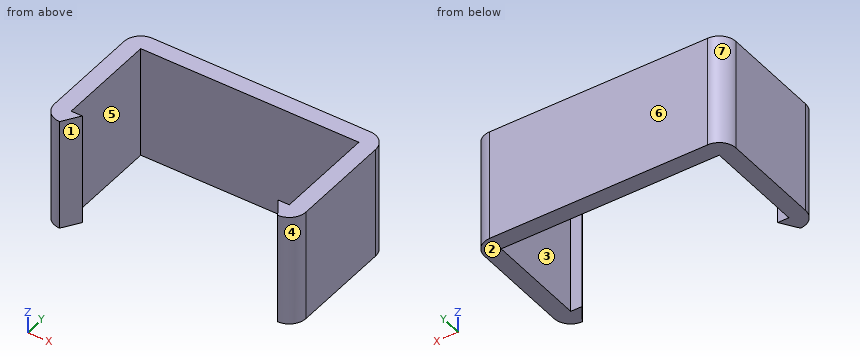
from build123d import *

# Parameters (mm, degrees)
F1_DEPTH = 20
F2_ANGLE = 270
F3_R     = 2.99999


# Not quite as in the source:
# - a fillet or chamfer is up to 0.001 mm smaller than in the source, because OpenCascade refuses the exact size


with BuildPart() as f1:
    # F0 (on Front) → F1 (new body)
    with BuildSketch(Plane.XZ):
        Polygon((22.5, 24), (-22.5, 24), (-22.5, 0), (-19.5, 0), (-17.5, 3), (-19.5, 3), (-19.5, 21), (19.5, 21), (19.5, 3), (17.5, 3), (19.5, 0), (22.5, 0), align=None)
    extrude(amount=F1_DEPTH)


with BuildPart() as f1_1:
    # F2: moved
    add(f1.part.rotate(Axis((0, -20, 24), (1, 0, 0)), F2_ANGLE))

    # F3 (radius 3 in the source; OpenCascade refuses exactly that, so slightly less here)
    f3_edges = [f1_1.edges().sort_by_distance(p)[0] for p in [
        (-22.5, -20, 14),
        (-22.5, -44, 14),
        (22.5, -44, 14),
        (22.5, -20, 14),
    ]]
    fillet(f3_edges, radius=F3_R)


solid = f1_1.part
Design review of the part built by this model. Coordinates are the model's own, in mm. Face numbers are marked on the shaded views. A direction names the side the tool comes from. Round coordinates to 2 decimals unless told otherwise and drop trailing zeros. Loops run counter-clockwise (first coordinate to the right, second up) from the corner with the lowest first, then second, coordinate; pieces in that order, holes last. Notation, with made-up numbers: (48.5, 86) -> (107.5, 86) arc R22 cw to (107.5, 122) -> close; hole circle Ø3 at (79.5, -39.75). An arc over 180 degrees is marked (long way). Use one line per item in the form item = value. Start each with the question number.
Q1. Draft analysis for pull direction X (two halves, no side actions). For the marked faces 4, 5, 6 and 7, state which applies: +X half, -X half, draft (parallel to the pull), parting line (faces both ways), or undercut.
Q2. For pin 1 Ø12 at (x, z) = (-2, 13) entering from -Y, flat-tipped, find the tip position at first contact; note if it passes through.
Q3. We need section A-A on y = -37. Give the boundary of the cut face in (x, z).
Q4. Wall thickness on line 1 along X through (y, z) = (-30.25, 23.25); line 2 along Y through (x, z) = (-13.5, 12); line 3 along X through (y, z) = (-42.25, 10): over which ranges is each line inside the solid? List them lowest first. Write a range as [from, to].
Q5. We need section C-C on x = -9. Give the boundary of the cut face in (y, z).
Q6. Machinability: for the marked faces 1, 2 and 3, which of the approach directions +Z, -Z, +X, -X, +Y, -Y give a long, thin tool a straight path to every point of the face, cutting with its end or side? Answer none if there is none.
Calculated:
q1.face_4 = +X half
q1.face_5 = undercut
q1.face_6 = draft
q1.face_7 = -X half
q2.pin_1 = -23
q3.outline = (-22.5, 4) -> (-19.5, 4) -> (-19.5, 24) -> (-22.5, 24) -> close; (19.5, 4) -> (22.5, 4) -> (22.5, 24) -> (19.5, 24) -> close
q4.line_1 = [-22.5, -19.5], [19.5, 22.5]
q4.line_2 = [-23, -20]
q4.line_3 = [-22.23, -18.33], [18.33, 22.23]
q5.outline = (-23, 4) -> (-20, 4) -> (-20, 24) -> (-23, 24) -> close
q6.face_1 = +Z, -Z, -Y
q6.face_2 = -Z, +X, -X, +Y, -Y
q6.face_3 = +Z, -Z
